from build123d import *

# Parameters (mm, degrees)
F0_R      = 500
F1_DEPTH  = 1300
F5_R      = 100
F6_DEPTH  = 809
F7_R      = 100
F8_DEPTH  = 384
F9_R      = 50
F10_DEPTH = 590


with BuildPart() as f1:
    # F0 (on Top) → F1 (new body)
    with BuildSketch(Plane.XY):
        Circle(F0_R)
    extrude(amount=F1_DEPTH)

    # F3 (on Front) → F4 (revolve)
    with BuildSketch(Plane.XZ):
        Polygon((0, 0), (0, -656.231495), (238.848731, 0), align=None)
    revolve(axis=Axis((0, 0, -328.115747), (0, 0, -1)))

    # F5 (on face) → F6 (cut)
    with BuildSketch(Plane(origin=(0, 0, 0), x_dir=(1, 0, 0), z_dir=(0, 0, -1))):
        Circle(F5_R)
    extrude(amount=F6_DEPTH, mode=Mode.SUBTRACT)

    # F7 (on face) → F8 (join)
    with BuildSketch(Plane(origin=(0, 0, 0), x_dir=(1, 0, 0), z_dir=(0, 0, -1))):
        Circle(F7_R)
    extrude(amount=F8_DEPTH)

    # F9 (on face) → F10 (join)
    with BuildSketch(Plane(origin=(0, 0, -384), x_dir=(1, 0, 0), z_dir=(0, 0, -1))):
        Circle(F9_R)
    extrude(amount=F10_DEPTH)


solid = f1.part
For this review, take the finished solid that the model builds, in its own axes (mm). A direction names the side the tool comes from. Coordinates: 2 decimals unless noted, no trailing zeros. Write each loop counter-clockwise with the first axis right and the second up, starting at its lowest first coordinate (ties: lowest second). Pieces come first, ordered by that corner, then holes. Notation, with made-up numbers: (18.25, 6.5) -> (46.25, 6.5) arc R21 ccw to (46.25, 43.5) -> close; hole circle Ø9 at (80.25, 64). An arc over 180 degrees is marked (long way). Write each question's results on one line, items separated by ' | '. Start each with the question number.
1) Insertion check: pin 1 (1.5 mm diameter, centred on y = 30.5, z = -541, fed in from -X); pin 2 (8 mm diameter, centred on x = -16, z = -384.5, fed in from -Y); pin 3 (2 mm diameter, centred on y = 84, z = 994.5, fed in from -X). Each pin has a flat end and moves straight along its axis. Give the tip position at first contact, or say it passes through.
2) Wall thickness on L1, parallel to Z at x = -216, y = -222.5; L2, parallel to X at y = -3, z = 362; L3, parallel to Y at x = -150, z = 905: over which ranges is each line inside the solid? List them lowest first. Write a range as [from, to].
3) Consider section A-A (y = 0). Write out the cut boundary in (x, z), plus the area to 3 significant figures.
4) Consider section C-C (z = 310). Write out the cut boundary in (x, y), plus the area to 3 significant figures.
5) Consider section D-D (y = 293.5). Write out the cut boundary in (x, z), plus the area to 3 significant figures.
6) For faces 1 (the face through (-499.516, 21.984, 640.9)), 2 (the face through (47.69, -15.02, -674.87)), list the 3-axis set-ups (+Z, -Z, +X, -X, +Y, -Y) from which the entire face can be reached by the end or side of a thin tool; tool diameter is ignored.
Geometry says:
1) pin 1: x = -40.19 | pin 2: y = -99.27 | pin 3: x = -493.06
2) L1: [0, 1300] | L2: [-499.99, 499.99] | L3: [-476.97, 476.97]
3) outline: (-500, 0) -> (-238.85, 0) -> (-100, -381.48) -> (-100, -384) -> (-50, -384) -> (-50, -974) -> (50, -974) -> (50, -384) -> (100, -384) -> (100, -381.48) -> (238.85, 0) -> (500, 0) -> (500, 1300) -> (-500, 1300) -> close | area: 1,490,000 mm^2
4) outline: circle Ø1000 at (0, 0) | area: 785,000 mm^2
5) outline: (-404.79, 0) -> (404.79, 0) -> (404.79, 1300) -> (-404.79, 1300) -> close | area: 1,050,000 mm^2
6) face 1: +Z, -Z | face 2: -Z
